Check sheet for the modelled part. Datum: model origin and axes. Units: mm. Face numbers are marked on the shaded views. A direction names the side the tool comes from. Coordinates: 2 decimals unless noted, no trailing zeros. Write each loop counter-clockwise with the first axis right and the second up, starting at its lowest first coordinate (ties: lowest second). Pieces come first, ordered by that corner, then holes. Notation, with made-up numbers: M 25,-9 L 66,-9 A23 cw 66,1 Z; hole C 20,60.5 d3. An arc over 180 degrees is marked long. Answer as CSV lines item,"result".
from build123d import *

# Parameters (mm, degrees)
BOSS_EXTRUDE1_DEPTH = 215.9
FILLET1_R           = 3.175
SKETCH2_R           = 3.175
CUT_EXTRUDE1_DEPTH  = 219.522128456
SKETCH3_R           = 3.175
CUT_EXTRUDE2_DEPTH  = 219.522128456
SKETCH4_R           = 3.175
CUT_EXTRUDE3_DEPTH  = 219.522128456
SKETCH5_R           = 3.175
CUT_EXTRUDE4_DEPTH  = 219.522128456


with BuildPart() as part:
    # Sketch1 → Boss-Extrude1 (new body)
    with BuildSketch(Plane(origin=(0, 0, 0), x_dir=(1, 0, 0), z_dir=(0, 1, 0))):
        Polygon((0, 0), (0, -25.4), (25.4, -25.4), (25.4, -22.225), (3.175, -22.225), (3.175, 0), align=None)
    extrude(amount=BOSS_EXTRUDE1_DEPTH)

    # Fillet1
    fillet1_edges = [part.edges().sort_by_distance(p)[0] for p in [
        (3.175, 107.95, 22.225),
    ]]
    fillet(fillet1_edges, radius=FILLET1_R)

    # Sketch2 → Cut-Extrude1 (cut, through all)
    with BuildSketch(Plane(origin=(0, 0, 22.225), x_dir=(-1, 0, 0), z_dir=(0, 0, -1))):
        with Locations((-15.875, 206.248)):
            Circle(SKETCH2_R)
    extrude(amount=-CUT_EXTRUDE1_DEPTH, mode=Mode.SUBTRACT)

    # Sketch3 → Cut-Extrude2 (cut, through all)
    with BuildSketch(Plane(origin=(0, 0, 22.225), x_dir=(-1, 0, 0), z_dir=(0, 0, -1))):
        with Locations((-15.875, 9.652)):
            Circle(SKETCH3_R)
    extrude(amount=-CUT_EXTRUDE2_DEPTH, mode=Mode.SUBTRACT)

    # Sketch4 → Cut-Extrude3 (cut, through all)
    with BuildSketch(Plane(origin=(3.175, 0, 0), x_dir=(0, 0, -1), z_dir=(1, 0, 0))):
        with Locations((-12.7, 206.375)):
            Circle(SKETCH4_R)
    extrude(amount=-CUT_EXTRUDE3_DEPTH, mode=Mode.SUBTRACT)

    # Sketch5 → Cut-Extrude4 (cut, through all)
    with BuildSketch(Plane(origin=(3.175, 0, 0), x_dir=(0, 0, -1), z_dir=(1, 0, 0))):
        with Locations((-12.7, 9.525)):
            Circle(SKETCH5_R)
    extrude(amount=-CUT_EXTRUDE4_DEPTH, mode=Mode.SUBTRACT)


solid = part.part
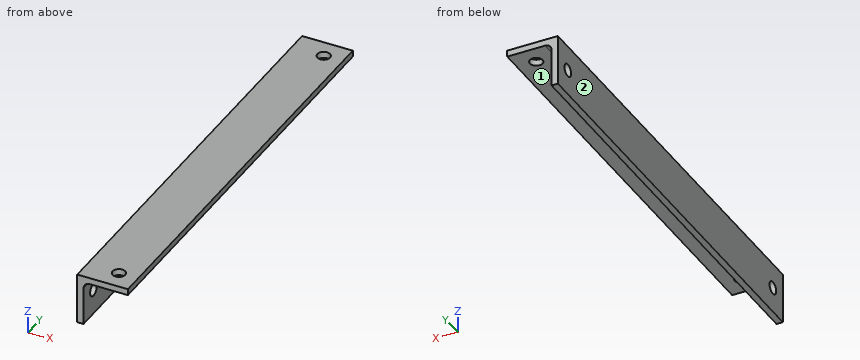
1) Section check A-A, the plane z = 12.7. Record the boundary of the cut face in (x, y) (3 decimals), plus the area to 3 significant figures.
Answer key:
outline,"M 0,0 L 3.175,0 L 3.175,6.35 L 0,6.35 Z; M 0,12.7 L 3.175,12.7 L 3.175,203.2 L 0,203.2 Z; M 0,209.55 L 3.175,209.55 L 3.175,215.9 L 0,215.9 Z"
area,"645 mm2"
2) Thickness scan on line 1 along Y through (x, z) = (2.25, 14); line 2 along Z through (x, y) = (19.75, 183) (3 decimals); line 3 along Y through (x, z) = (1, 11). Record the ranges inside material, lowest first.
Answer key:
line 1,"y = 0 to 6.63, 12.42 to 203.48, 209.27 to 215.9"
line 2,"z = 22.225 to 25.4"
line 3,"y = 0 to 6.84, 12.21 to 203.69, 209.06 to 215.9"
3) Depth check by flat-ended pin: P1, Ø4, axis at x = 15.875, y = 9.652, coming from the +Z side; P2, Ø8, axis at y = 122, z = 16.5, coming from the +X side; P3, Ø1, axis at x = 6, y = 167.5, coming from the -Z side; P4, Ø5.5, axis at x = 12, y = 112.5, coming from the -Z side (3 decimals). Enter the tip coordinate at first touch or a pass-through.
Answer key:
P1,"passes through"
P2,"stops at x = 3.53"
P3,"stops at z = 22.11"
P4,"stops at z = 22.225"
4) Section check B-B, the plane y = 182. Record the boundary of the cut face in (x, z) (3 decimals).
Answer key:
outline,"M 0,0 L 3.175,0 L 3.175,19.05 A3.175 cw 6.35,22.225 L 25.4,22.225 L 25.4,25.4 L 0,25.4 Z"
5) Section check C-C, the plane z = 3.75. Record the boundary of the cut face in (x, y) (3 decimals), plus the area to 3 significant figures.
Answer key:
outline,"M 0,0 L 3.175,0 L 3.175,215.9 L 0,215.9 Z"
area,"685 mm2"
6) Tool access check on the marked faces 1 and 2. Record the directions out of +Z, -Z, +X, -X, +Y, -Y that give a thin tool (end or side, any length) a straight path to the whole face; none if there is none.
Answer key:
face 1,"-Z, +X, +Y, -Y"
face 2,"+Z, -Z, -X, +Y, -Y"
7) Section check D-D, the plane x = 10. Record the boundary of the cut face in (y, z) (3 decimals).
Answer key:
outline,"M 0,22.225 L 215.9,22.225 L 215.9,25.4 L 0,25.4 Z"
